The drawing under review shows one solid part. Ordinate dimensions are in mm from its lowest x, y, z. A direction names the side the tool comes from. Give positions to 0.01 mm unless a question says otherwise; leave off trailing zeros. Write each loop counter-clockwise with the first axis right and the second up, starting at its lowest first coordinate (ties: lowest second). Pieces come first, ordered by that corner, then holes.
Q1. We need section B-B (x = 61). Write out the cut boundary in (y, z), then the cut area to 3 significant figures.
Q2. We need section D-D (x = 183). Write out the cut boundary in (y, z).
Q3. For line 1 (Y direction, x = 100.5, z = 17.25); line 2 (Y direction, x = 40, z = 26.55); line 3 (X direction, y = 9, z = 6.5), list the stretches that pass through material, from the lowest coordinate up.
Q4. We need section C-C (y = 22). Write out the cut boundary in (x, z).
Q5. Machinability: for the marked faces 4, 5 and 6, which of the approach directions +Z, -Z, +X, -X, +Y, -Y give a long, thin tool a straight path to every point of the face, cutting with its end or side? Answer none if there is none.
Q6. We need section A-A (z = 14.75). Write out the cut boundary in (x, y), then the cut area to 3 significant figures.
Q7. Insertion check: P1, Ø6, axis at y = 3.5, z = 17.5, coming from the +X side; P2, Ø14, axis at x = 16, y = 10, coming from the -Z side; P3, Ø3, axis at x = 135, y = 19, coming from the +Z side; P4, Ø2.5, axis at x = 40, y = 14, coming from the -Z side. Each pin has a flat end and moves straight along its axis. Give the tip position at first contact, or say it passes through.
Q8. Mouldability with a two-part tool opening along X and no side actions: class the marked faces 1, 2 and 3 as released by +X, released by -X, zero draft, split by the parting line, or undercut.
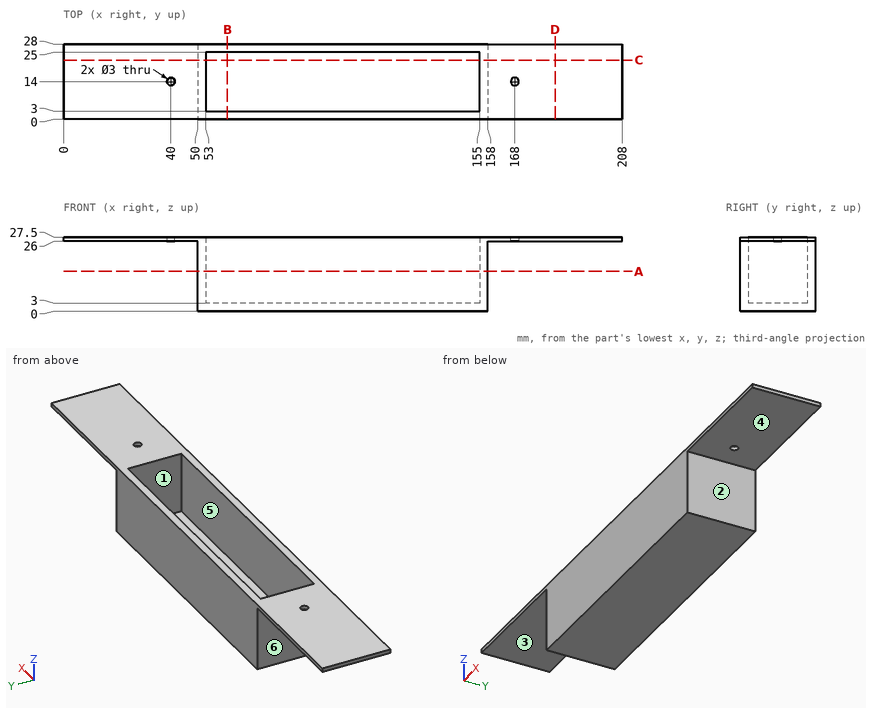
Computed:
1. outline: (0, 0) - (28, 0) - (28, 27.5) - (25, 27.5) - (25, 3) - (3, 3) - (3, 27.5) - (0, 27.5) - close
1. area: 231 mm2
2. outline: (0, 26) - (28, 26) - (28, 27.5) - (0, 27.5) - close
3. line 1: y = 0 to 3, 25 to 28
3. line 2: y = 0 to 12.5, 15.5 to 28
3. line 3: x = 50 to 53, 155 to 158
4. outline: (0, 26) - (50, 26) - (50, 0) - (158, 0) - (158, 26) - (208, 26) - (208, 27.5) - (155, 27.5) - (155, 3) - (53, 3) - (53, 27.5) - (0, 27.5) - close
5. face 4: -Z, +X, +Y, -Y
5. face 5: +Z
5. face 6: -Z, -X, +Y, -Y
6. outline: (50, 0) - (158, 0) - (158, 28) - (50, 28) - close; hole (53, 3) - (155, 3) - (155, 25) - (53, 25) - close
6. area: 780 mm2
7. P1: stops at x = 158
7. P2: stops at z = 26
7. P3: stops at z = 3
7. P4: passes through
8. face 1: undercut
8. face 2: released by +X
8. face 3: zero draft
